Verification items for the finished model (mm, model axes). A direction names the side the tool comes from. Give positions to 0.01 mm unless a question says otherwise; leave off trailing zeros. Order: outer loops, then holes, each group sorted by start corner. A loop starts at its lowest first (then second) coordinate and runs counter-clockwise, first axis right, second up. Notation, with made-up numbers: (-26, 82.25) -> (-20, 82.25) arc R11 ccw to (-20, 103.25) -> close; hole circle Ø10 at (-11, 52). An arc over 180 degrees is marked (long way). Write each question's results on one line, items separated by ' | '. Start each with the question number.
1. Mould release check, pull along Z, two halves, no side actions. Record for faces 1 (the face through (118, 0, 20)), 2 (the face through (50, -1, 22)), 3 (the face through (41.22, 19.503, 21.972)), 4 (the face through (1.97, -1.08, 4.88)): +Z half, -Z half, draft (parallel to the pull), parting line (faces both ways), or undercut.
2. Set-up check for faces 5 (the face through (3, 17.4, 22)), 6 (the face through (18.91, -14.33, 23.01)), 7 (the face through (213, -5, 22)), 8 (the face through (217.95, 8, 22)), 9 (the face through (140, -10, 22)): record each of +Z, -Z, +X, -X, +Y, -Y from which the full face is reachable in a straight line by a thin tool's end or side.
3. Cross-section at C-C, the plane z = 9.5. Enter the section's corners in (x, y) (3 decimals), then the cut area to 3 significant figures.
4. Cross-section at A-A, the plane z = 0. Enter the section's corners in (x, y).
5. Cross-section at B-B, the plane x = 106. Enter the section's corners in (y, z).
6. Depth check by flat-ended pin: pin 1 Ø1.3 at (x, y) = (226, -8) entering from -Z; pin 2 Ø4 at (x, y) = (72.5, -6) entering from -Z; pin 3 Ø2 at (x, z) = (221, 22) entering from -Y; pin 4 Ø6 at (y, z) = (-5.5, 1.5) entering from +X. Enter the tip coordinate at first touch or a pass-through.
7. Material ranges on L1, parallel to Y at x = 20.75, z = 21.05; L2, parallel to Z at x = 117, y = -8.5; L3, parallel to X at y = -10.5, z = -9.5, recorded low to high. Write a range as from..to.
Autodesk Inventor part; units mm, degrees
ref_plane "YZ Plane" through (0, 0, 0) normal (1, 0, 0) x (0, 1, 0)
ref_plane "XZ Plane" through (0, 0, 0) normal (0, 1, 0) x (-1, 0, 0)
ref_plane "XY Plane" through (0, 0, 0) normal (0, 0, 1) x (1, 0, 0)
sketch "スケッチ1" plane through (0, 0, 0) normal (1, 0, 0) x (0, 1, 0)
  circle A0 centre (0, 0) radius 10
  circle A1 centre (0, -10) radius 1.35
  circle A2 centre (8.6603, 5) radius 1.35
  circle A3 centre (-8.6603, 5) radius 1.35
  circle A4 centre (0, 0) radius 5
  line L0 (0, 0) -> (0, 50)
  circle A5 centre (0, 50) radius 22.5
  circle A6 centre (0, 0) radius 14
  line L1 (-14, 0) -> (-22.5, 50)
  line L2 (14, 0) -> (22.5, 50)
  line L3 (0, -14) -> (-11.62, -14)
  line L4 (-11.62, -14) -> (-14, 0)
  line L5 (0, -14) -> (11.62, -14)
  line L6 (11.62, -14) -> (14, 0)
  line L7 (0, 20) -> (-17.4, 20)
  line L8 (0, 20) -> (17.4, 20)
  dimension "d0" = 20
  dimension "d1" = 2.7
  dimension "d4" = 360
  dimension "d6" = 10
  dimension "d7" = 50
  dimension "d8" = 45
  dimension "d9" = 28
extrude "押し出し1" add sketch "スケッチ1" along normal blind 4 contours A0 A1 A3 A2 | A6 L6 L4 | A6 L1 L7 L0 | L0 L8 L2 A6 | L6 L5 A6 | A6 L3 L4
sketch "スケッチ2" plane through (0, -17.4, 20) normal (0, 0, 1) x (1, 0, 0)
  line L0 (0, 17.4) -> (30, 17.4)
  circle A0 centre (30, 17.4) radius 22.5
  circle A1 centre (30, 17.4) radius 18.5
  circle A2 centre (30, 17.4) radius 14.25
  circle A3 centre (48.5, 17.4) radius 1.35
  circle A4 centre (20.75, 33.4215) radius 1.35
  circle A5 centre (20.75, 1.3785) radius 1.35
  line L1 (0, 29.02) -> (0, 34.8)
  line L2 (0, 0) -> (0, 5.78)
  line L3 (0, 34.8) -> (0, 0)
  line L4 (4, 29.02) -> (4, 34.8)
  line L5 (4, 34.8) -> (7, 34.8)
  line L6 (7, 34.8) -> (30, 39.9)
  line L7 (4, 0) -> (4, 5.78)
  line L8 (4, 0) -> (7, 0)
  line L9 (7, 0) -> (30, -5.1)
  line L10 (4, 0) -> (0, 0)
  line L11 (0, 34.8) -> (4, 34.8)
  line L12 (0, 0) -> (0, 34.8)
  line L13 (0, 34.8) -> (4, 34.8)
  dimension "d14" = 37
  dimension "d12" = 30
  dimension "d13" = 45
  dimension "d15" = 28.5
  dimension "d16" = 2.7
  dimension "d19" = 360
  dimension "d21" = 3
  dimension "d22" = 3
extrude "押し出し2" add sketch "スケッチ2" along normal blind 4 contours L3 L1 L11 L5 L6 A0 L0 | L0 A0 L9 L8 L10 L2 L3 | A1 A4 A3 A5 | A0 L6 L9
fillet "フィレット1" radius 3 2 edges at (4, 0, 20) (0, 0, 24)
fillet "フィレット2" radius 3 2 edges at (2, -11.62, -14) (2, 11.62, -14)
sketch "スケッチ7" plane through (0, -17.4, 24) normal (0, 0, 1) x (1, 0, 0)
  circle A0 centre (30, 17.4) radius 14.25
  line L0 (30, 17.4) -> (182.95, 17.4)
  line L1 (30, 17.4) -> (182.95, 17.4) construction
  circle A1 centre (182.95, 17.4) radius 3.5
  circle A2 centre (182.95, 17.4) radius 10
  line L2 (182.95, 27.4) -> (50.1556, 27.4)
  arc A3 (30, -5.1) -> (30, 39.9) centre (30, 17.4) ccw
  line L3 (182.95, 27.4) -> (315.7444, 27.4) construction
  line L4 (182.95, 7.4) -> (50.1556, 7.4)
  point P0 (0, 17.4)
  dimension "d55" = 152.95
  dimension "d56" = 0
  dimension "d57" = 7
  dimension "d58" = 20
  dimension "d59" = 180
extrude "押し出し7" add sketch "スケッチ7" against normal blind 4 contours A3 L2 A2 L0 | L0 A2 L4 A3 | A2
sketch "スケッチ8" plane through (0, -17.4, 24) normal (0, 0, 1) x (1, 0, 0)
  circle A0 centre (20.75, 33.4215) radius 1.35
  circle A1 centre (20.75, 33.4215) radius 2.5
  circle A2 centre (48.5, 17.4) radius 1.35
  circle A3 centre (48.5, 17.4) radius 2.5
  circle A4 centre (20.75, 1.3785) radius 1.35
  circle A5 centre (20.75, 1.3785) radius 2.5
  point P0 (0, 17.4)
  dimension "d63" = 5
  dimension "d64" = 5
  dimension "d65" = 5
extrude "押し出し8" cut sketch "スケッチ8" against normal blind 2 contours A0 | A1 | A3 | A4 | A5
fillet "フィレット4" radius 2 1 edges at (50.1556, 10, 22)
sketch "スケッチ12" plane through (0, -17.4, 24) normal (0, 0, 1) x (1, 0, 0)
  circle A0 centre (48.5, 17.4) radius 2.5
  circle A1 centre (20.75, 1.3785) radius 2.5
  circle A2 centre (20.75, 33.4215) radius 2.5
  circle A3 centre (182.95, 17.4) radius 3.5
  line L0 (3, 0) -> (3, 34.8)
  line L1 (3, 0) -> (7, 0)
  line L2 (7, 0) -> (30, -5.1)
  arc A4 (30, -5.1) -> (50.1556, 7.4) centre (30, 17.4) ccw
  line L3 (50.1556, 7.4) -> (182.95, 7.4)
  arc A5 (182.95, 7.4) -> (182.95, 27.4) centre (182.95, 17.4) ccw
  line L4 (182.95, 27.4) -> (51.36, 27.4)
  arc A6 (49.6163, 28.4204) -> (51.36, 27.4) centre (51.36, 29.4) ccw
  arc A7 (49.6163, 28.4204) -> (30, 39.9) centre (30, 17.4) ccw
  line L5 (30, 39.9) -> (7, 34.8)
  line L6 (7, 34.8) -> (3, 34.8)
  circle A8 centre (30, 17.4) radius 14.25
  line L7 (182.95, 7.4) -> (232.95, 7.4)
  line L8 (182.95, 27.4) -> (232.95, 27.4)
  line L9 (232.95, 27.4) -> (232.95, 7.4)
  point P0 (0, 17.4)
  dimension "d92" = 50
  dimension "d93" = 50
extrude "押し出し12" add sketch "スケッチ12" against normal blind 4 contours A5 L8 L9 L7
sketch "スケッチ14" plane through (0, -17.4, 24) normal (0, 0, 1) x (1, 0, 0)
  circle A0 centre (30, 17.4) radius 14.25
  line L0 (232.95, 27.4) -> (51.36, 27.4)
  arc A1 (49.6163, 28.4204) -> (51.36, 27.4) centre (51.36, 29.4) ccw
  arc A2 (49.6163, 28.4204) -> (30, 39.9) centre (30, 17.4) ccw
  line L1 (30, 39.9) -> (7, 34.8)
  line L2 (7, 34.8) -> (3, 34.8)
  line L3 (3, 0) -> (3, 34.8)
  line L4 (3, 0) -> (7, 0)
  line L5 (7, 0) -> (30, -5.1)
  arc A3 (30, -5.1) -> (50.1556, 7.4) centre (30, 17.4) ccw
  line L6 (50.1556, 7.4) -> (232.95, 7.4)
  circle A4 centre (182.95, 17.4) radius 3.5
  circle A5 centre (20.75, 33.4215) radius 2.5
  circle A6 centre (20.75, 1.3785) radius 2.5
  circle A7 centre (48.5, 17.4) radius 2.5
  line L7 (197.95, 27.4) -> (197.95, 12.4)
  line L8 (197.95, 12.4) -> (227.95, 12.4)
  line L9 (227.95, 12.4) -> (227.95, 22.4)
  line L10 (227.95, 22.4) -> (217.95, 22.4)
  line L11 (217.95, 22.4) -> (217.95, 27.4)
  line L12 (232.95, 7.4) -> (232.95, 27.4)
  point P0 (0, 17.4)
  dimension "d110" = 10
  dimension "d113" = 30
  dimension "d118" = 5
  dimension "d119" = 5
  dimension "d120" = 5
  dimension "d121" = 5
extrude "押し出し14" cut sketch "スケッチ14" against normal blind 4 contours L11 L10 L9 L8 L7 L0
fillet "フィレット8" radius 1 6 edges at (197.95, -5, 22) (232.95, 10, 22) (232.95, -10, 22) (217.95, 5, 22) (227.95, -5, 22) (227.95, 5, 22)
sketch "スケッチ15" plane through (0, -17.4, 24) normal (0, 0, 1) x (1, 0, 0)
  circle A0 centre (226, 9.4) radius 1.1
  circle A1 centre (220, 9.4) radius 1.1
  line L0 (0, 0) -> (0, 5.3555)
  line L1 (0, 0) -> (240, 0)
  line L2 (50.1556, 7.4) -> (231.95, 7.4)
  line L3 (0, 0) -> (240, 0) construction
  point P0 (0, 17.4)
  dimension "d123" = 2.2
  dimension "d124" = 2.2
  dimension "d130" = 240
  dimension "d131" = 0
  dimension "d132" = 9.4
  dimension "d133" = 9.4
  dimension "d134" = 6
extrude "押し出し15" cut sketch "スケッチ15" against normal blind 10
properties part number "motor_holder_8-5" material "ABS プラスチック"
Results below:
1) face 1: -Z half | face 2: +Z half | face 3: draft | face 4: undercut
2) face 5: +Z, -Z, -X, +Y | face 6: +Z | face 7: +Z, -Z | face 8: +Z, -Z, +Y | face 9: +Z, -Z, +X, -Y
3) outline: (0, -15.615) -> (4, -15.615) -> (4, 15.615) -> (0, 15.615) -> close | area: 125 mm²
4) outline: (0, -14) -> (4, -14) -> (4, -5) -> (0, -5) -> close; (0, 5) -> (4, 5) -> (4, 14) -> (0, 14) -> close
5) outline: (-10, 20) -> (10, 20) -> (10, 24) -> (-10, 24) -> close
6) pin 1: passes through | pin 2: stops at z = 20 | pin 3: stops at y = -10 | pin 4: stops at x = 4
7) L1: y = -20.45..-17.37, -14.67..-10.84, 10.84..14.67, 17.37..20.45 | L2: z = 20..24 | L3: x = 0..4
